The model under review builds one solid part; all positions refer to its coordinate system, in mm. A direction names the side the tool comes from. Round coordinates to 2 decimals unless told otherwise and drop trailing zeros. Loops run counter-clockwise (first coordinate to the right, second up) from the corner with the lowest first, then second, coordinate; pieces in that order, holes last. Notation, with made-up numbers: M 1.5,76.5 L 41.5,76.5 A20 ccw 41.5,113.5 Z; hole C 71.5,14.25 d8. An arc over 180 degrees is marked long. Return JSON: item names as keys, results as strings. Group by question number.
Q1. For faces 1 (the face through (6, 2.5, -9)), 2 (the face through (4.89, 1.93, -2.76)), list the 3-axis set-ups (+Z, -Z, +X, -X, +Y, -Y) from which the entire face can be reached by the end or side of a thin tool; tool diameter is ignored.
Q2. Consider section A-A (y = 0.9). State the section outline as (x, z) points, and give its area (3 significant figures).
Q3. Draft analysis for pull direction X (two halves, no side actions). For faces 3 (the face through (12, 2, -1)), 4 (the face through (6, 3, -4.55)), 5 (the face through (4.8, 1.2, -11.1)), state which applies: pulls with the +X half, pulls with the -X half, needs draft (parallel to the pull), parting line crosses it, or undercut.
Q4. Clearance check with flat-ended pins moving along their axes: pin 1 Ø4 at (x, z) = (9.5, -6) entering from +Y; pin 2 Ø3 at (x, z) = (6, -8.5) entering from +Y; pin 3 Ø0.6 at (x, y) = (7.5, 3.5) entering from -Z; pin 4 Ø1.8 at (x, z) = (6, -12) entering from -Y. State where each tip first meets the part, or that it passes through.
Q5. Consider section D-D (y = 3.05). State the section outline as (x, z) points, and give its area (3 significant figures).
Q6. To check wall thickness, follow line 1 along Z through (x, y) = (6, 0.5); line 2 along X through (y, z) = (3.05, -1.75); line 3 along Y through (x, z) = (11.25, -5.75). State the ranges of each line that lie inside material, in increasing order.
Q7. Consider section C-C (z = -1.75). State the section outline as (x, y) points, and give its area (3 significant figures).
Q8. Consider section B-B (x = 6). State the section outline as (y, z) points, and give its area (3 significant figures).
from build123d import *

# Parameters (mm, degrees)
SKETCH1_R           = 1.5
BOSS_EXTRUDE1_DEPTH = 2.5
FILLET2_R           = 2
BOSS_EXTRUDE2_DEPTH = 1.3
SKETCH3_R           = 1.5
CUT_EXTRUDE1_DEPTH  = 3.8


with BuildPart() as part:
    # Sketch1 → Boss-Extrude1 (new body)
    with BuildSketch(Plane(origin=(0, 0, 0), x_dir=(1, 0, 0), z_dir=(0, 1, 0))):
        with BuildLine():
            Line((2.079207921, 12.792079208), (0, 2.5))
            Line((0, 2.5), (0, 0))
            Line((0, 0), (12, 0))
            Line((12, 0), (12, 2.5))
            Line((12, 2.5), (9.920792079, 12.792079208))
            ThreePointArc((9.920792079, 12.792079208), (6, 16), (2.079207921, 12.792079208))
        make_face()
        with Locations((6, 12)):
            Circle(SKETCH1_R, mode=Mode.SUBTRACT)
    extrude(amount=BOSS_EXTRUDE1_DEPTH)

    # Fillet2
    fillet2_edges = [part.edges().sort_by_distance(p)[0] for p in [
        (0, 1.25, -2.5),
        (12, 1.25, -2.5),
    ]]
    fillet(fillet2_edges, radius=FILLET2_R)

    # Sketch2 → Boss-Extrude2 (add)
    with BuildSketch(Plane(origin=(0, 2.5, 0), x_dir=(1, 0, 0), z_dir=(0, 1, 0))):
        Polygon((0.414141414, 4.55), (11.585858586, 4.55), (11.96039604, 2.696039604), (12, 2.3), (12, 0), (0, 0), (0, 2.3), (0.03960396, 2.696039604), align=None)
    extrude(amount=BOSS_EXTRUDE2_DEPTH)

    # Sketch3 → Cut-Extrude1 (cut)
    with BuildSketch(Plane(origin=(0, 3.8, 0), x_dir=(1, 0, 0), z_dir=(0, 1, 0))):
        with Locations((6, 1.75)):
            Circle(SKETCH3_R)
    extrude(amount=-CUT_EXTRUDE1_DEPTH, mode=Mode.SUBTRACT)


solid = part.part
Values:
{
 "1": {"face 1": "-Z, +X, -X, +Y", "face 2": "+Y, -Y"},
 "2": {"outline": "M 0,-2.3 A2 ccw 0.04,-2.7 L 2.08,-12.79 A4 ccw 9.92,-12.79 L 11.96,-2.7 A2 ccw 12,-2.3 L 12,0 L 0,0 Z; hole C 6,-12 d3; hole C 6,-1.75 d3", "area": "137 mm2"},
 "3": {"face 3": "pulls with the +X half", "face 4": "needs draft", "face 5": "undercut"},
 "4": {"pin 1": "stops at y = 3.8", "pin 2": "stops at y = 2.5", "pin 3": "stops at z = -4.55", "pin 4": "passes through"},
 "5": {"outline": "M 0,-2.3 L 0.04,-2.7 L 0.41,-4.55 L 11.59,-4.55 L 11.96,-2.7 L 12,-2.3 L 12,0 L 0,0 Z; hole C 6,-1.75 d3", "area": "46.7 mm2"},
 "6": {"line 1": "z = -16 to -13.5, -10.5 to -3.25, -0.25 to 0", "line 2": "x = 0 to 4.5, 7.5 to 12", "line 3": "y = 0 to 2.5"},
 "7": {"outline": "M 0,0 L 4.5,0 L 4.5,3.8 L 0,3.8 Z; M 7.5,0 L 12,0 L 12,3.8 L 7.5,3.8 Z", "area": "34.2 mm2"},
 "8": {"outline": "M 0,-16 L 2.5,-16 L 2.5,-13.5 L 0,-13.5 Z; M 0,-10.5 L 2.5,-10.5 L 2.5,-4.55 L 3.8,-4.55 L 3.8,-3.25 L 0,-3.25 Z; M 0,-0.25 L 3.8,-0.25 L 3.8,0 L 0,0 Z", "area": "27.0 mm2"}
}
